Part model, mm, in its own coordinate system. Round coordinates to 2 decimals unless told otherwise and drop trailing zeros. Loops run counter-clockwise (first coordinate to the right, second up) from the corner with the lowest first, then second, coordinate; pieces in that order, holes last.
(1) Cut at C-C on y = 0.85. Count the separate pieces of the cut face and the enclosed holes in it, then the cut area to 3 significant figures.
(2) Cut at B-B on x = 476. List the corners of the cut face in (y, z), then the cut area to 3 significant figures.
(3) Cut at A-A on x = -476.5. List the corners of the cut face in (y, z).
(4) Probe probe 1 along Z at (x, y) = (456.5, 1.35); probe 2 along Z at (x, y) = (-497.5, 2.45); probe 3 along X at (y, z) = (1.2, -166). List the from-to ranges inside material, lowest first.
from build123d import *

# Parameters (mm, degrees)
SKETCH1_W           = 96.800297879
SKETCH1_H           = 14.479859902
SKETCH1_H_2         = 14.476525066
SKETCH1_W_2         = 96.796963042
SKETCH1_H_3         = 14.526547613
SKETCH1_H_4         = 14.51987794
BOSS_EXTRUDE1_DEPTH = 3


with BuildPart() as part:
    # Sketch1 → Boss-Extrude1 (new body)
    with BuildSketch(Plane(origin=(0, 0, 0), x_dir=(1, 0, 0), z_dir=(0, 1, 0))):
        Polygon((686.70035272, 239.579653428), (686.70035272, 225.059775488), (692.749746056, 225.059775488), (692.749746056, 210.533227875), (686.70035272, 210.533227875), (686.70035272, 181.491804577), (672.178807362, 181.491804577), (672.178807362, 210.533227875), (666.129414026, 210.533227875), (666.129414026, 225.059775488), (672.178807362, 225.059775488), (672.178807362, 239.579653428), (612.025027325, 239.579653428), (612.025027325, 196.600281152), (571.723528724, 196.600281152), (571.723528724, 239.579653428), (367.346408951, 239.579653428), (367.346408951, 196.600281152), (327.043242933, 196.600281152), (327.043242933, 239.579653428), (251.100679683, 239.579653428), (251.100679683, 225.059775488), (257.150073019, 225.059775488), (257.150073019, 210.533227875), (251.100679683, 210.533227875), (251.100679683, 181.491804577), (236.579134325, 181.491804577), (236.579134325, 210.533227875), (230.529740989, 210.533227875), (230.529740989, 225.059775488), (236.579134325, 225.059775488), (236.579134325, 239.579653428), (166.747658885, 239.579653428), (166.747658885, 196.600281152), (126.446160285, 196.600281152), (126.446160285, 239.579653428), (-77.92929207, 239.579653428), (-77.92929207, 196.600281152), (-118.232458088, 196.600281152), (-118.232458088, 239.579653428), (-203.85271674, 239.579653428), (-203.85271674, 225.059775488), (-197.803323405, 225.059775488), (-197.803323405, 210.533227875), (-203.85271674, 210.533227875), (-203.85271674, 181.491804577), (-218.374262098, 181.491804577), (-218.374262098, 210.533227875), (-224.425322852, 210.533227875), (-224.425322852, 225.059775488), (-218.374262098, 225.059775488), (-218.374262098, 239.579653428), (-326.669741249, 239.579653428), (-326.669741249, 196.600281152), (-366.97123985, 196.600281152), (-366.97123985, 239.579653428), (-571.348359623, 239.579653428), (-571.348359623, 196.600281152), (-611.649858223, 196.600281152), (-611.649858223, 239.579653428), (-780.777756631, 239.579653428), (-780.777756631, -239.579653428), (-611.649858223, -239.579653428), (-611.649858223, -196.323489726), (-571.348359623, -196.323489726), (-571.348359623, -239.579653428), (-366.97123985, -239.579653428), (-366.97123985, -196.323489726), (-326.669741249, -196.323489726), (-326.669741249, -239.579653428), (-218.374262098, -239.579653428), (-218.374262098, -225.059775488), (-224.425322852, -225.059775488), (-224.425322852, -210.539897548), (-218.374262098, -210.539897548), (-218.374262098, -181.500141668), (-203.85271674, -181.500141668), (-203.85271674, -210.539897548), (-197.803323405, -210.539897548), (-197.803323405, -225.059775488), (-203.85271674, -225.059775488), (-203.85271674, -239.579653428), (-118.232458088, -239.579653428), (-118.232458088, -196.323489726), (-77.92929207, -196.323489726), (-77.92929207, -239.579653428), (126.446160285, -239.579653428), (126.446160285, -196.323489726), (166.747658885, -196.323489726), (166.747658885, -239.579653428), (236.582469161, -239.579653428), (236.582469161, -225.059775488), (230.533075826, -225.059775488), (230.533075826, -210.539897548), (236.582469161, -210.539897548), (236.582469161, -181.500141668), (251.102347101, -181.500141668), (251.102347101, -210.539897548), (257.151740437, -210.539897548), (257.151740437, -225.059775488), (251.102347101, -225.059775488), (251.102347101, -239.579653428), (327.046577769, -239.579653428), (327.046577769, -196.323489726), (367.349743788, -196.323489726), (367.349743788, -239.579653428), (571.716859051, -239.579653428), (571.716859051, -196.323489726), (612.02002507, -196.323489726), (612.02002507, -239.579653428), (672.172137689, -239.579653428), (672.172137689, -225.059775488), (666.121076935, -225.059775488), (666.121076935, -210.539897548), (672.172137689, -210.539897548), (672.172137689, -181.500141668), (686.692015629, -181.500141668), (686.692015629, -210.539897548), (692.741408964, -210.539897548), (692.741408964, -225.059775488), (686.692015629, -225.059775488), (686.692015629, -239.579653428), (780.777756631, -239.579653428), (780.777756631, 239.579653428), align=None)
        Polygon((-421.022269168, -166.9502502), (-517.822567047, -166.9502502), (-517.822567047, -152.470390298), (-421.023936586, -152.470390298), align=None, mode=Mode.SUBTRACT)
        Polygon((-421.022269168, 152.497068989), (-517.822567047, 152.497068989), (-517.822567047, 166.973594055), (-421.023936586, 166.973594055), align=None, mode=Mode.SUBTRACT)
        with Locations((24.258434108, -159.710320249)):
            Rectangle(SKETCH1_W, SKETCH1_H, mode=Mode.SUBTRACT)
        with Locations((24.258434108, 159.735331522)):
            Rectangle(SKETCH1_W, SKETCH1_H_2, mode=Mode.SUBTRACT)
        with Locations((469.537469965, -159.686976394)):
            Rectangle(SKETCH1_W_2, SKETCH1_H_3, mode=Mode.SUBTRACT)
        with Locations((469.537469965, 159.757007959)):
            Rectangle(SKETCH1_W_2, SKETCH1_H_4, mode=Mode.SUBTRACT)
    extrude(amount=BOSS_EXTRUDE1_DEPTH)


solid = part.part
Final values:
1. separate pieces: 1
1. enclosed holes: 6
1. area: 713,000 mm2
2. outline: (0, -239.58) - (3, -239.58) - (3, -167.02) - (0, -167.02) - close; (0, -152.5) - (3, -152.5) - (3, 152.42) - (0, 152.42) - close; (0, 166.95) - (3, 166.95) - (3, 239.58) - (0, 239.58) - close
2. area: 1,350 mm2
3. outline: (0, -239.58) - (3, -239.58) - (3, -166.97) - (0, -166.97) - close; (0, -152.5) - (3, -152.5) - (3, 152.47) - (0, 152.47) - close; (0, 166.95) - (3, 166.95) - (3, 239.58) - (0, 239.58) - close
4. probe 1: z = -239.58 to -167.02, -152.5 to 152.42, 166.95 to 239.58
4. probe 2: z = -239.58 to -166.97, -152.5 to 152.47, 166.95 to 239.58
4. probe 3: x = -780.78 to -517.82, -421.02 to -24.14, 72.66 to 421.14, 517.94 to 780.78
